Autodesk Inventor part; units mm, degrees
ref_plane "YZ Plane" through (0, 0, 0) normal (1, 0, 0) x (0, 1, 0)
ref_plane "XZ Plane" through (0, 0, 0) normal (0, 1, 0) x (-1, 0, 0)
ref_plane "XY Plane" through (0, 0, 0) normal (0, 0, 1) x (1, 0, 0)
sketch "Sketch1" plane through (0, 0, 0) normal (0, 0, 1) x (1, 0, 0)
  line L0 (5.9771, 0) -> (28.2021, 0)
  line L1 (28.2021, 0) -> (28.2021, 3.175)
  line L2 (28.2021, 3.175) -> (5.9771, 3.175)
  line L3 (2.8021, 6.35) -> (2.8021, 25.4)
  line L4 (5.9771, 28.575) -> (28.2021, 28.575)
  line L5 (28.2021, 28.575) -> (28.2021, 31.75)
  line L6 (28.2021, 31.75) -> (5.9771, 31.75)
  line L7 (-0.3729, 25.4) -> (-0.3729, 6.35)
  arc A0 (5.9771, 28.575) -> (2.8021, 25.4) centre (5.9771, 25.4) ccw
  arc A1 (2.8021, 6.35) -> (5.9771, 3.175) centre (5.9771, 6.35) ccw
  arc A2 (5.9771, 31.75) -> (-0.3729, 25.4) centre (5.9771, 25.4) ccw
  arc A3 (-0.3729, 6.35) -> (5.9771, 0) centre (5.9771, 6.35) ccw
  point P0 (0, 0)
  point P1 (-0.3729, 0)
  point P2 (2.8021, 3.175)
  point P3 (2.8021, 28.575)
  dimension "d0" = 28.575
  dimension "d1" = 3.175
  dimension "d2" = 25.4
  dimension "d3" = 25.4
  dimension "d4" = 3.175
  dimension "d5" = 3.175
  dimension "d6" = 6.35
extrude "Extrusion1" add sketch "Sketch1" against normal blind 889
sketch "Sketch2" plane through (-0.3729, 6.35, 0) normal (-1, 0, 0) x (0, 0, 1)
  line L0 (0, 19.05) -> (-889, 19.05)
  line L1 (-228.6, 0) -> (-228.6, 7.9375)
  arc A0 (-228.6, 11.1125) -> (-228.6, 7.9375) centre (-228.6, 9.525) ccw
  line L2 (-228.6, 11.1125) -> (-228.6, 19.05)
  line L3 (-228.6, 19.05) -> (-889, 19.05)
  line L4 (-889, 0) -> (-889, 19.05)
  line L5 (-889, 0) -> (-228.6, 0)
  circle A1 centre (-552.45, 11.43) radius 4.826
  circle A2 centre (-501.65, 11.43) radius 4.826
  circle A3 centre (-387.35, 11.43) radius 4.826
  circle A4 centre (-336.55, 11.43) radius 4.826
  circle A5 centre (-444.5, 7.62) radius 4.826
  circle A6 centre (-730.25, 11.43) radius 4.826
  circle A7 centre (-781.05, 11.43) radius 4.826
  line L6 (0, 25.4) -> (-889, 25.4) construction
  circle A8 centre (-133.35, 11.43) radius 4.826
  circle A9 centre (-82.55, 11.43) radius 4.826
  point P0 (0, -6.35)
  point P1 (-254, 0.852)
  dimension "d10" = 7.62
  dimension "d11" = 3.81
  dimension "d14" = 254
hole "Hole1" at (-0.3729, 17.78, -781.05) at (-0.3729, 17.78, -730.25) at (-0.3729, 17.78, -552.45) at (-0.3729, 17.78, -501.65) at (-0.3729, 13.97, -444.5) at (-0.3729, 17.78, -387.35) at (-0.3729, 17.78, -336.55) at (-0.3729, 17.78, -133.35) at (-0.3729, 17.78, -82.55) direction (1, 0, 0) diameter 9.652 end through all
hole "Hole2" at (-0.3729, 15.875, -228.6) direction (1, 0, 0) diameter 3.175 end through all
sketch "Sketch3" plane through (5.9771, 31.75, 0) normal (0, 1, 0) x (1, 0, 0)
  line L0 (22.225, 889) -> (0, 889)
  line L1 (22.225, 0) -> (22.225, 889)
  point P0 (-5.9771, 0)
  point P1 (9.525, 876.3)
  dimension "d34" = 12.7
  dimension "d35" = 12.7
hole "Hole3" at (15.5021, 31.75, -876.3) direction (0, -1, 0) diameter 6.5278 end through all
pattern_linear "Rectangular Pattern1" count 35 spacing 25.4 along (0, 0, 1) of "Hole3"
sketch "Sketch4" plane through (5.9771, 31.75, 0) normal (0, 1, 0) x (1, 0, 0)
  circle A0 centre (9.525, 12.7) radius 3.2639
  circle A1 centre (9.525, 38.1) radius 3.2639
  circle A2 centre (9.525, 63.5) radius 3.2639
  circle A3 centre (9.525, 88.9) radius 3.2639
  circle A4 centre (9.525, 114.3) radius 3.2639
  circle A5 centre (9.525, 139.7) radius 3.2639
  circle A6 centre (9.525, 165.1) radius 3.2639
  circle A7 centre (9.525, 190.5) radius 3.2639
  line L0 (22.225, 0) -> (-13.6032, 0)
  line L1 (-13.6032, 0) -> (-13.6032, 685.8)
  line L2 (-13.6032, 685.8) -> (22.225, 685.8)
  line L3 (22.225, 685.8) -> (22.225, 0)
  point P0 (-5.9771, 0)
  dimension "d46" = 685.8
extrude "Extrusion2" cut sketch "Sketch4" against normal blind 38.1
properties part number "chassis 9 inch"
Geometry check sheet. Reference: the model listing, model coordinates, mm. A direction names the side the tool comes from. Coordinates: 2 decimals unless noted, no trailing zeros. Order: outer loops, then holes, each group sorted by start corner. A loop starts at its lowest first (then second) coordinate and runs counter-clockwise, first axis right, second up.
Item 1: Section check C-C (z = -768). Enter the section's corners in (x, y) (3 decimals), plus the area to 3 significant figures.
Item 2: Mould release check, pull along Y, two halves, no side actions. Record for faces 3 (the flat face through (2, 15, -685.8)), 4 (the cylindrical face through (3.71, 4.13, -785.98)), 5 (the cylindrical face through (1.237, 19.628, -725.792)), 6 (the cylindrical face through (1.54, 29.94, -785.98)): released by +Y, released by -Y, zero draft, split by the parting line, or undercut.
Item 3: Section check A-A (x = 24.5). Enter the section's corners in (y, z) (3 decimals), plus the area to 3 significant figures.
Item 4: Depth check by flat-ended pin: pin 1 (9.5 mm diameter, centred on y = 19.5, z = -759.5, fed in from +X). Enter the tip coordinate at first touch or a pass-through.
Item 5: Tool access check on faces 1 (the cylindrical face through (3.76, 27.67, -785.98)), 2 (the cylindrical face through (14.522, 1.565, -796.987)). Record the directions out of +Z, -Z, +X, -X, +Y, -Y that give a thin tool (end or side, any length) a straight path to the whole face; none if there is none.
Item 6: Scan lines: line 1 along Z through (x, y) = (1.7, 17.78); line 2 along Y through (x, z) = (26.5, -708) (3 decimals); line 3 along X through (y, z) = (6, -823.5). Record each from-to range of solid material in increasing order.
Item 7: Section check B-B (z = -825.5). Enter the section's corners in (x, y) (3 decimals), plus the area to 3 significant figures.
Check sheet entries:
1. outline: (-0.373, 6.35) arc R6.35 ccw to (5.977, 0) - (28.202, 0) - (28.202, 3.175) - (5.977, 3.175) arc R3.175 cw to (2.802, 6.35) - (2.802, 25.4) arc R3.175 cw to (5.977, 28.575) - (28.202, 28.575) - (28.202, 31.75) - (5.977, 31.75) arc R6.35 ccw to (-0.373, 25.4) - close
1. area: 249 mm2
2. face 3: zero draft
2. face 4: undercut
2. face 5: undercut
2. face 6: released by +Y
3. outline: (0, -889) - (3.175, -889) - (3.175, -685.8) - (0, -685.8) - close; (28.575, -889) - (31.75, -889) - (31.75, -685.8) - (28.575, -685.8) - close
3. area: 1,290 mm2
4. pin 1: stops at x = 2.8
5. face 1: +Z, -Z, +X
5. face 2: +Y, -Y
6. line 1: z = -889 to -785.88, -776.22 to -735.08, -725.42 to -685.8
6. line 2: y = 0 to 3.175, 28.575 to 31.75
6. line 3: x = -0.36 to 2.82
7. outline: (-0.373, 6.35) arc R6.35 ccw to (5.977, 0) - (12.238, 0) - (12.238, 3.175) - (5.977, 3.175) arc R3.175 cw to (2.802, 6.35) - (2.802, 25.4) arc R3.175 cw to (5.977, 28.575) - (12.238, 28.575) - (12.238, 31.75) - (5.977, 31.75) arc R6.35 ccw to (-0.373, 25.4) - close; (18.766, 0) - (28.202, 0) - (28.202, 3.175) - (18.766, 3.175) - close; (18.766, 28.575) - (28.202, 28.575) - (28.202, 31.75) - (18.766, 31.75) - close
7. area: 208 mm2
